Here's how the part is built. I have some questions about the finished solid (model axes, mm). Round coordinates to 2 decimals unless told otherwise and drop trailing zeros. Use one line per item in the form item = value. Start each with the question number.
1. I want a section at A-A, the plane y = -5. State how many separate pieces and enclosed holes the cut face has, plus the area to 3 significant figures.
2. We'd pull the mould along X, two halves only. Please class faces 1 (the flat face through (-23.4, 0, 23.4)), 2 (the cylindrical face through (74.41, -4.94, -22.41)): +X half, -X half, draft (parallel to the pull), parting line (faces both ways), or undercut.
3. Will these pins go through, and if not, where does the flat tip stop? pin 1 (2 mm diameter, centred on x = -38, y = -8.5, fed in from -Z); pin 2 (1 mm diameter, centred on x = 2.5, y = -3, fed in from +Z); pin 3 (1.5 mm diameter, centred on y = -5, z = 39.5, fed in from -X).
4. If I drill on line 1 along X through (y, z) = (-4, 0); line 2 along Z through (x, y) = (-85.5, -0.25); line 3 along X through (y, z) = (-1.75, -17.5), over which ranges is the centre line in solid material (lowest first)?
```python
from build123d import *

# Parameters (mm, degrees)
F0_R     = 7.5
F1_DEPTH = 10
F2_SIZE2 = 1
F2_SIZE  = 1
F3_SIZE2 = 1
F3_SIZE  = 1
F4_SIZE2 = 2
F4_SIZE  = 2
F5_SIZE2 = 2
F5_SIZE  = 2
F6_SIZE2 = 1
F6_SIZE  = 1
F7_SIZE2 = 1
F7_SIZE  = 1


with BuildPart() as f1:
    # F0 (on Front) → F1 (new body)
    with BuildSketch(Plane.XZ):
        with BuildLine():
            ThreePointArc((0, 100), (-70.710678, -70.710678), (100, 0))
            ThreePointArc((100, 0), (70.710678, 70.710678), (0, 100))
        make_face()
        with Locations((-22.743852, -81.900654)):
            Circle(F0_R, mode=Mode.SUBTRACT)
        with Locations((-81.811651, -23.00498)):
            Circle(F0_R, mode=Mode.SUBTRACT)
        with Locations((23.093983, -82.072779)):
            Circle(F0_R, mode=Mode.SUBTRACT)
        with Locations((81.900654, -22.743852)):
            Circle(F0_R, mode=Mode.SUBTRACT)
        with Locations((-81.900654, 22.743852)):
            Circle(F0_R, mode=Mode.SUBTRACT)
        with BuildLine():
            ThreePointArc((-15.243852, 81.900654), (-16.773045, 77.361992), (-20.737042, 74.674126))
            ThreePointArc((-20.737042, 74.674126), (-28.714659, 86.439317), (-15.243852, 81.900654))
        make_face(mode=Mode.SUBTRACT)
        with BuildLine():
            ThreePointArc((-8.161029, 29.387882), (-4.118228, 30.220692), (0, 30.5))
            ThreePointArc((0, 30.5), (4.118228, 30.220692), (8.161029, 29.387882))
            ThreePointArc((8.161029, 29.387882), (24.281283, 18.457229), (30.5, 0))
            ThreePointArc((30.5, 0), (-18.457229, -24.281283), (-8.161029, 29.387882))
        make_face(mode=Mode.SUBTRACT)
        with Locations((82.161782, 22.832855)):
            Circle(F0_R, mode=Mode.SUBTRACT)
        with BuildLine():
            ThreePointArc((30.243852, 81.900654), (27.282515, 75.929847), (20.737042, 74.674126))
            ThreePointArc((20.737042, 74.674126), (18.205189, 87.871462), (30.243852, 81.900654))
        make_face(mode=Mode.SUBTRACT)
    extrude(amount=F1_DEPTH)

    # F2
    f2_edges = [f1.edges().sort_by_distance(p)[0] for p in [
        (-100, 0, 0),
    ]]
    chamfer(f2_edges, length=F2_SIZE, length2=F2_SIZE2)

    # F3
    f3_edges = [f1.edges().sort_by_distance(p)[0] for p in [
        (-100, -10, 0),
    ]]
    chamfer(f3_edges, length=F3_SIZE, length2=F3_SIZE2)

    # F4
    f4_edges = [f1.edges().sort_by_distance(p)[0] for p in [
        (8.161029, 0, -29.387882),
    ]]
    chamfer(f4_edges, length=F4_SIZE, length2=F4_SIZE2)

    # F5
    f5_edges = [f1.edges().sort_by_distance(p)[0] for p in [
        (8.161029, -10, -29.387882),
    ]]
    chamfer(f5_edges, length=F5_SIZE, length2=F5_SIZE2)

    # F6
    f6_edges = [f1.edges().sort_by_distance(p)[0] for p in [
        (15.243852, 0, 81.900654),
        (-30.243852, 0, 81.900654),
        (-89.400654, 0, 22.743852),
        (-89.311651, 0, -23.00498),
        (-30.243852, 0, -81.900654),
        (15.593983, 0, -82.072779),
        (74.400654, 0, -22.743852),
        (74.661782, 0, 22.832855),
    ]]
    chamfer(f6_edges, length=F6_SIZE, length2=F6_SIZE2)

    # F7
    f7_edges = [f1.edges().sort_by_distance(p)[0] for p in [
        (-30.243852, -10, 81.900654),
        (15.243852, -10, 81.900654),
        (74.661782, -10, 22.832855),
        (74.400654, -10, -22.743852),
        (15.593983, -10, -82.072779),
        (-30.243852, -10, -81.900654),
        (-89.400654, -10, 22.743852),
        (-89.311651, -10, -23.00498),
    ]]
    chamfer(f7_edges, length=F7_SIZE, length2=F7_SIZE2)


solid = f1.part
```
Model answer:
q1.separate_pieces = 1
q1.enclosed_holes = 9
q1.area = 27,100 mm2
q2.face_1 = draft
q2.face_2 = undercut
q3.pin_1 = -92.9
q3.pin_2 = 99.98
q3.pin_3 = -92.19
q4.line_1 = -100 to -30.5, 30.5 to 100
q4.line_2 = -50.4 to -30.38, -15.63 to 15.32, 30.17 to 50.4
q4.line_3 = -98.46 to -86.91, -76.72 to -25.28, 25.28 to 76.54, 87.26 to 98.46
